```python
from build123d import *

# Parameters (mm, degrees)
ESQUISSE1_W               = 98
ESQUISSE1_H               = 60
BOSS_EXTRU_1_DEPTH        = 1.6
ESQUISSE2_R               = 1.6
ENL_V_MAT_EXTRU_1_DEPTH   = 58.476603936
SYM_TRIE2_COPY_1_SKETCH_R = 1.6
SYM_TRIE2_COPY_1_DEPTH    = 58.476603936
ESQUISSE3_W               = 5
ESQUISSE3_H               = 12
ESQUISSE3_W_2             = 10
ESQUISSE3_H_2             = 6
ESQUISSE3_H_3             = 2.54
BOSS_EXTRU_2_DEPTH        = 12


with BuildPart() as part:
    # Esquisse1 → Boss.-Extru.1 (new body)
    with BuildSketch(Plane.XY):
        Rectangle(ESQUISSE1_W, ESQUISSE1_H)
    extrude(amount=BOSS_EXTRU_1_DEPTH)

    # Esquisse2 → Enlèv. mat.-Extru.1 (cut, through all)
    with BuildSketch(Plane.XY.offset(1.6)):
        with Locations((-46.5, 27.5)):
            Circle(ESQUISSE2_R)
    enl_v_mat_extru_1 = extrude(amount=-ENL_V_MAT_EXTRU_1_DEPTH, mode=Mode.SUBTRACT)

    # Symétrie1: Enlèv. mat.-Extru.1 across plane
    add(enl_v_mat_extru_1.mirror(Plane.ZX), mode=Mode.SUBTRACT)

    # Symétrie2: Enlèv. mat.-Extru.1 across plane
    add(enl_v_mat_extru_1.mirror(Plane(origin=(0, 0, 0), x_dir=(0, 0, 1), z_dir=(1, 0, 0))), mode=Mode.SUBTRACT)

    # Symétrie2 copy 1 sketch → Symétrie2 copy 1 (cut, through all)
    with BuildSketch(Plane(origin=(0, 0, 1.6), x_dir=(-1, 0, 0), z_dir=(0, 0, 1))):
        with Locations((-46.5, 27.5)):
            Circle(SYM_TRIE2_COPY_1_SKETCH_R)
    extrude(amount=-SYM_TRIE2_COPY_1_DEPTH, mode=Mode.SUBTRACT)

    # Esquisse3 → Boss.-Extru.2 (add)
    with BuildSketch(Plane.XY.offset(1.6)):
        with Locations((35.7, -9)):
            Rectangle(ESQUISSE3_W, ESQUISSE3_H)
        with Locations((23, -17)):
            Rectangle(ESQUISSE3_W_2, ESQUISSE3_H_2)
        with Locations((-13.5, 4.73)):
            Rectangle(ESQUISSE3_W, ESQUISSE3_H_3)
    extrude(amount=BOSS_EXTRU_2_DEPTH)


solid = part.part
```
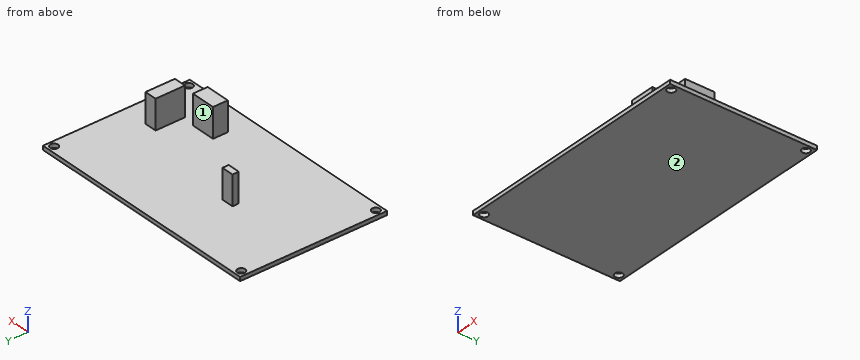
Verification items for the finished model (mm, model axes). Face numbers are marked on the shaded views. A direction names the side the tool comes from. Coordinates: 2 decimals unless noted, no trailing zeros. Write each loop counter-clockwise with the first axis right and the second up, starting at its lowest first coordinate (ties: lowest second). Pieces come first, ordered by that corner, then holes. Notation, with made-up numbers: M -1.5,47 L 43.5,47 A22 cw 43.5,64 Z; hole C 16.5,89.5 d4. An arc over 180 degrees is marked long. One line per item, written item: value.
Item 1: Section check A-A, the plane y = 27.5. Record the boundary of the cut face in (x, z), plus the area to 3 significant figures.
Check sheet entries:
outline: M -49,0 L -48.1,0 L -48.1,1.6 L -49,1.6 Z; M -44.9,0 L 44.9,0 L 44.9,1.6 L -44.9,1.6 Z; M 48.1,0 L 49,0 L 49,1.6 L 48.1,1.6 Z
area: 147 mm^2
Item 2: Scan lines: line 1 along X through (y, z) = (-27.5, 0.45); line 2 along Y through (x, z) = (-46.5, 1); line 3 along Z through (x, y) = (41.5, 13). Record each from-to range of solid material in increasing order.
Check sheet entries:
line 1: x = -49 to -48.1, -44.9 to 44.9, 48.1 to 49
line 2: y = -30 to -29.1, -25.9 to 25.9, 29.1 to 30
line 3: z = 0 to 1.6
Item 3: Access from +Z, -Z, +X, -X, +Y, -Y to the whole of each face (thin tool, end or side, straight path). Record for the marked faces 1 and 2.
Check sheet entries:
face 1: +Z, -X, +Y
face 2: -Z, +X, -X, +Y, -Y
Item 4: Section check C-C, the plane y = -4. Record the boundary of the cut face in (x, z), plus the area to 3 significant figures.
Check sheet entries:
outline: M -49,0 L 49,0 L 49,1.6 L 38.2,1.6 L 38.2,13.6 L 33.2,13.6 L 33.2,1.6 L -49,1.6 Z
area: 217 mm^2
Item 5: Section check D-D, the plane x = -27. Record the boundary of the cut face in (y, z), plus the area to 3 significant figures.
Check sheet entries:
outline: M -30,0 L 30,0 L 30,1.6 L -30,1.6 Z
area: 96.0 mm^2
Item 6: Gauge pin test, flat ends, axial feed: pin 1 Ø5 at (y, z) = (-18, 5.5) entering from -X; pin 2 Ø1.5 at (x, z) = (-14.5, 6) entering from -Y; pin 3 Ø5 at (x, y) = (-46.5, 27.5) entering from +Z. Record the tip position at first contact, or that the pin passes through.
Check sheet entries:
pin 1: stops at x = 18
pin 2: stops at y = 3.46
pin 3: stops at z = 1.6
Item 7: Section check B-B, the plane x = -46.5. Record the boundary of the cut face in (y, z).
Check sheet entries:
outline: M -30,0 L -29.1,0 L -29.1,1.6 L -30,1.6 Z; M -25.9,0 L 25.9,0 L 25.9,1.6 L -25.9,1.6 Z; M 29.1,0 L 30,0 L 30,1.6 L 29.1,1.6 Z
